Can you work these out from the model? Positions are in its coordinate system, mm. A direction names the side the tool comes from. Coordinates: 2 decimals unless noted, no trailing zeros. Loops run counter-clockwise (first coordinate to the right, second up) from the corner with the lowest first, then second, coordinate; pieces in that order, holes last.
```python
from build123d import *

# Parameters (mm, degrees)
BOX123_W          = 1
BOX123_H          = 35
BOX123_DEPTH      = 2
BOX126_W          = 2.5
BOX126_H          = 36
BOX126_DEPTH      = 4
BOX128_W          = 64
BOX128_H          = 1
BOX128_DEPTH      = 2
BOX131_W          = 59
BOX131_H          = 2
BOX131_DEPTH      = 2
BOX125_W          = 1
BOX125_H          = 35
BOX125_DEPTH      = 2
CYLINDER055_R     = 8
CYLINDER055_DEPTH = 2
CYLINDER054_R     = 8
CYLINDER054_DEPTH = 2
CYLINDER057_R     = 6
CYLINDER057_DEPTH = 2
CYLINDER056_R     = 6
CYLINDER056_DEPTH = 2
BOX130_W          = 20
BOX130_H          = 12
BOX130_DEPTH      = 2
BOX129_W          = 59
BOX129_H          = 36
BOX129_DEPTH      = 2
BOX122_W          = 2.5
BOX122_H          = 36
BOX122_DEPTH      = 4
FILLET026_R       = 1.9
FILLET027_R       = 9


with BuildPart() as cube113:
    # Box123 → Box123 (new body)
    with BuildSketch(Plane(origin=(27.5, -4, -15), x_dir=(1, 0, 0), z_dir=(0, 0, 1))):
        with Locations((0.5, 17.5)):
            Rectangle(BOX123_W, BOX123_H)
    extrude(amount=BOX123_DEPTH)


with BuildPart() as cube116:
    # Box126 → Box126 (new body)
    with BuildSketch(Plane(origin=(89, -5, -19), x_dir=(1, 0, 0), z_dir=(0, 0, 1))):
        with Locations((1.25, 18)):
            Rectangle(BOX126_W, BOX126_H)
    extrude(amount=BOX126_DEPTH)


with BuildPart() as cube118:
    # Box128 → Box128 (new body)
    with BuildSketch(Plane(origin=(27.5, -5, -15), x_dir=(1, 0, 0), z_dir=(0, 0, 1))):
        with Locations((32, 0.5)):
            Rectangle(BOX128_W, BOX128_H)
    extrude(amount=BOX128_DEPTH)


with BuildPart() as cube121:
    # Box131 → Box131 (new body)
    with BuildSketch(Plane(origin=(30, -5, -17), x_dir=(1, 0, 0), z_dir=(0, 0, 1))):
        with Locations((29.5, 1)):
            Rectangle(BOX131_W, BOX131_H)
    extrude(amount=BOX131_DEPTH)


with BuildPart() as cube115:
    # Box125 → Box125 (new body)
    with BuildSketch(Plane(origin=(90.5, -4, -15), x_dir=(1, 0, 0), z_dir=(0, 0, 1))):
        with Locations((0.5, 17.5)):
            Rectangle(BOX125_W, BOX125_H)
    extrude(amount=BOX125_DEPTH)


with BuildPart() as cylinder136:
    # Cylinder055 → Cylinder055 (new body)
    with BuildSketch(Plane(origin=(80, 20, -19), x_dir=(1, 0, 0), z_dir=(0, 0, 1))):
        Circle(CYLINDER055_R)
    extrude(amount=CYLINDER055_DEPTH)


with BuildPart() as cylinder135:
    # Cylinder054 → Cylinder054 (new body)
    with BuildSketch(Plane(origin=(39, 20, -19), x_dir=(1, 0, 0), z_dir=(0, 0, 1))):
        Circle(CYLINDER054_R)
    extrude(amount=CYLINDER054_DEPTH)


with BuildPart() as cylinder138:
    # Cylinder057 → Cylinder057 (new body)
    with BuildSketch(Plane(origin=(39, 4, -19), x_dir=(1, 0, 0), z_dir=(0, 0, 1))):
        Circle(CYLINDER057_R)
    extrude(amount=CYLINDER057_DEPTH)


with BuildPart() as cylinder137:
    # Cylinder056 → Cylinder056 (new body)
    with BuildSketch(Plane(origin=(80, 4, -19), x_dir=(1, 0, 0), z_dir=(0, 0, 1))):
        Circle(CYLINDER056_R)
    extrude(amount=CYLINDER056_DEPTH)


with BuildPart() as cube120:
    # Box130 → Box130 (new body)
    with BuildSketch(Plane(origin=(49.5, 19, -19), x_dir=(1, 0, 0), z_dir=(0, 0, 1))):
        with Locations((10, 6)):
            Rectangle(BOX130_W, BOX130_H)
    extrude(amount=BOX130_DEPTH)


with BuildPart() as cut081:
    # Box129 → Box129 (new body)
    with BuildSketch(Plane(origin=(30, -5, -19), x_dir=(1, 0, 0), z_dir=(0, 0, 1))):
        with Locations((29.5, 18)):
            Rectangle(BOX129_W, BOX129_H)
    extrude(amount=BOX129_DEPTH)

    # Cut077: cut Cube120
    add(cube120.part, mode=Mode.SUBTRACT)

    # Cut078: cut Cylinder137
    add(cylinder137.part, mode=Mode.SUBTRACT)

    # Cut079: cut Cylinder138
    add(cylinder138.part, mode=Mode.SUBTRACT)

    # Cut080: cut Cylinder135
    add(cylinder135.part, mode=Mode.SUBTRACT)

    # Cut081: cut Cylinder136
    add(cylinder136.part, mode=Mode.SUBTRACT)


with BuildPart() as fillet027:
    # Box122 → Box122 (new body)
    with BuildSketch(Plane(origin=(27.5, -5, -19), x_dir=(1, 0, 0), z_dir=(0, 0, 1))):
        with Locations((1.25, 18)):
            Rectangle(BOX122_W, BOX122_H)
    extrude(amount=BOX122_DEPTH)

    # Fusion045: union Cube113, Cube116, Cube118, Cube121, Cube115, Cut081
    add(cube113.part)
    add(cube116.part)
    add(cube118.part)
    add(cube121.part)
    add(cube115.part)
    add(cut081.part)

    # Fillet026
    fillet026_edges = [fillet027.edges().sort_by_distance(p)[0] for p in [
        (27.5, 13, -19),
        (91.5, 13, -19),
    ]]
    fillet(fillet026_edges, radius=FILLET026_R)

    # Fillet027
    fillet027_edges = [fillet027.edges().sort_by_distance(p)[0] for p in [
        (49.5, 31, -18),
        (69.5, 31, -18),
    ]]
    fillet(fillet027_edges, radius=FILLET027_R)


solid = fillet027.part
```
(1) If I drill on probe 1 along Y at (x, z) = (80, -17.7); probe 2 along X at (y, z) = (2.5, -16.45); probe 3 along Z at (x, y) = (50.5, 15.5), over which ranges is the centre line in solid material (lowest first)?
Check values:
probe 1: y = -5 to -2, 10 to 12, 28 to 31
probe 2: x = 27.5 to 30, 89 to 91.5
probe 3: z = -19 to -17
(2) I want a section at C-C on z = -15.65. Write out the boundary of the cut face in (x, y).
Check values:
outline: (27.5, -5) - (91.5, -5) - (91.5, 31) - (89, 31) - (89, -3) - (30, -3) - (30, 31) - (27.5, 31) - close
(3) If we mould it in two halves opening along Y, with no side actions, what happens to faces 1 (the cylindrical face through (33, 4, -18)), 2 (the cylindrical face through (74, 4, -18)), 3 (the cylindrical face through (46.934, 28.294, -17.986)), 4 (the flat face through (59, 10, -17))? For each: released by +Y, released by -Y, zero draft, split by the parting line, or undercut.
Check values:
face 1: undercut
face 2: undercut
face 3: released by +Y
face 4: zero draft
(4) I'm going to push flat-ended pins straight in: pin 1 (1 mm diameter, centred on y = 20.5, z = -18, fed in from -X); pin 2 (2 mm diameter, centred on x = 56.5, z = -18.5, fed in from +Y); pin 3 (2 mm diameter, centred on x = 65.5, z = -14.5, fed in from +Y). Where does each tip first touch, or does it pass through?
Check values:
pin 1: stops at x = 27.54
pin 2: stops at y = 19
pin 3: stops at y = -3
(5) I want a section at D-D on y = 6. Write out the boundary of the cut face in (x, z), then the cut area to 3 significant figures.
Check values:
outline: (27.5, -17.1) arc R1.9 ccw to (29.4, -19) - (33.34, -19) - (33.34, -17) - (30, -17) - (30, -15) - (28.5, -15) - (28.5, -13) - (27.5, -13) - close; (44.66, -19) - (74.34, -19) - (74.34, -17) - (44.66, -17) - close; (85.66, -19) - (89.6, -19) arc R1.9 ccw to (91.5, -17.1) - (91.5, -13) - (90.5, -13) - (90.5, -15) - (89, -15) - (89, -17) - (85.66, -17) - close
area: 95.2 mm2
(6) I want a section at B-B on x = 80. Write out the boundary of the cut face in (y, z).
Check values:
outline: (-5, -19) - (-2, -19) - (-2, -17) - (-3, -17) - (-3, -15) - (-4, -15) - (-4, -13) - (-5, -13) - close; (10, -19) - (12, -19) - (12, -17) - (10, -17) - close; (28, -19) - (31, -19) - (31, -17) - (28, -17) - close
(7) I want a section at A-A on y = 20. Write out the boundary of the cut face in (x, z).
Check values:
outline: (27.5, -17.1) arc R1.9 ccw to (29.4, -19) - (31, -19) - (31, -17) - (30, -17) - (30, -15) - (28.5, -15) - (28.5, -13) - (27.5, -13) - close; (47, -19) - (49.5, -19) - (49.5, -17) - (47, -17) - close; (69.5, -19) - (72, -19) - (72, -17) - (69.5, -17) - close; (88, -19) - (89.6, -19) arc R1.9 ccw to (91.5, -17.1) - (91.5, -13) - (90.5, -13) - (90.5, -15) - (89, -15) - (89, -17) - (88, -17) - close
(8) Which directions (+Z, -Z, +X, -X, +Y, -Y) give clear straight access to the entire face, cutting with the end or side of a thin tool? Please do faces 5 (the cylindrical face through (90.958, 13.252, -18.429)), 6 (the cylindrical face through (72.206, 28.434, -17.986)), 7 (the flat face through (30, 14, -16)).
Check values:
face 5: -Z, +X, +Y, -Y
face 6: +Z, -Z, +Y
face 7: +Z, +Y
